```python
from build123d import *

# Parameters (mm, degrees)
SKETCH1_W           = 210
SKETCH1_H           = 40
BOSS_EXTRUDE1_DEPTH = 40
SKETCH2_R           = 6
BOSS_EXTRUDE2_DEPTH = 100


with BuildPart() as part:
    # Sketch1 → Boss-Extrude1 (new body)
    with BuildSketch(Plane.XY):
        with Locations((-105, 0)):
            Rectangle(SKETCH1_W, SKETCH1_H)
    extrude(amount=BOSS_EXTRUDE1_DEPTH)

    # Sketch2 → Boss-Extrude2 (add)
    with BuildSketch(Plane.ZY.offset(210)):
        with Locations((20, 0)):
            Circle(SKETCH2_R)
    extrude(amount=BOSS_EXTRUDE2_DEPTH)

    # Mirror1: part across plane


with BuildPart() as part_1:
    add(part.part)
    add(part.part.mirror(Plane(origin=(0, 20, 40), x_dir=(0, 0, 1), z_dir=(-1, 0, 0))))


solid = part_1.part
```
Work out the finished part from the listing and answer in its coordinate system (mm). A direction names the side the tool comes from. Coordinates: 2 decimals unless noted, no trailing zeros. Loops run counter-clockwise (first coordinate to the right, second up) from the corner with the lowest first, then second, coordinate; pieces in that order, holes last.
1) For faces 1 (the flat face through (210, -5, 15)), 2 (the flat face through (-210, -5, 15)), 3 (the flat face through (310, 0, 20)), determine the directions among +Z, -Z, +X, -X, +Y, -Y from which every point of the face is accessible in a straight line to the end or side of a thin tool.
Results:
face 1: +X
face 2: -X
face 3: +Z, -Z, +X, +Y, -Y
2) Section C-C (x = 261) is taken. Give the vertices of the cut face in (y, z).
Results:
outline: circle Ø12 at (0, 20)
3) Consider probe 1 along Z at (x, y) = (252, -1); probe 2 along X at (y, z) = (-18, 2); probe 3 along Y at (x, z) = (-266.5, 22.5). Determine where each line is inside the solid, lowest interval first.
Results:
probe 1: z = 14.08 to 25.92
probe 2: x = -210 to 210
probe 3: y = -5.45 to 5.45
4) Section A-A (y = 0) is taken. Give the vertices of the cut face in (x, z), plus the area to 3 significant figures.
Results:
outline: (-310, 14) - (-210, 14) - (-210, 0) - (210, 0) - (210, 14) - (310, 14) - (310, 26) - (210, 26) - (210, 40) - (-210, 40) - (-210, 26) - (-310, 26) - close
area: 19,200 mm2
5) Flat-ended cylindrical pins translate along their axes: pin 1 (5 mm diameter, centred on x = -165, y = 3.5, fed in from -Z); pin 2 (1 mm diameter, centred on y = -16, z = 20.5, fed in from -X); pin 3 (8 mm diameter, centred on x = 214.5, z = 18.5, fed in from -Y). Find the tip coordinate at first contact, or state that the pin passes through.
Results:
pin 1: stops at z = 0
pin 2: stops at x = -210
pin 3: stops at y = -6
6) Section B-B (z = 20) is taken. Give the vertices of the cut face in (x, y), plus the area to 3 significant figures.
Results:
outline: (-310, -6) - (-210, -6) - (-210, -20) - (210, -20) - (210, -6) - (310, -6) - (310, 6) - (210, 6) - (210, 20) - (-210, 20) - (-210, 6) - (-310, 6) - close
area: 19,200 mm2
